Input: dimensioned drawing with shaded views. Units: mm. Origin: part minimum x, y, z. Round coordinates to 2 decimals unless told otherwise and drop trailing zeros. Loops run counter-clockwise (first coordinate to the right, second up) from the corner with the lowest first, then second, coordinate; pieces in that order, holes last. Notation, with made-up numbers: (52, -12) - (77, -12) arc R19 ccw to (77, 17) - close; hole circle Ø8 at (18.25, 67.25). An arc over 180 degrees is marked (long way). One line per question, with ' | ' between items.
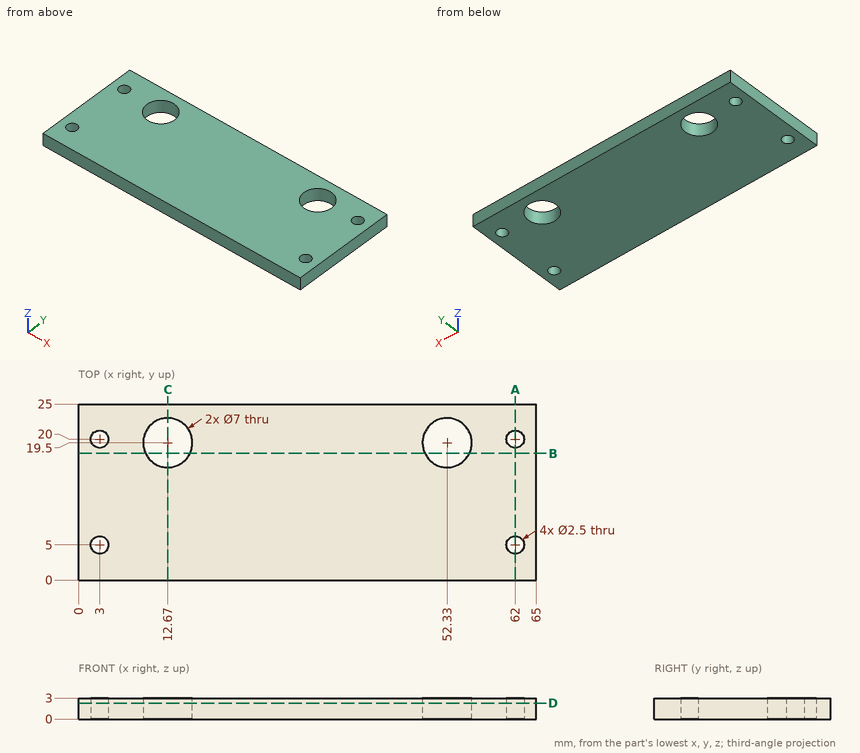
1. Material intervals for probe 1 along Y at (x, z) = (62, 1.55); probe 2 along Y at (x, z) = (12.67, 0.8); probe 3 along X at (y, z) = (16.5, 0.95), sorted ascending.
Worked out:
probe 1: y = 0 to 3.75, 6.25 to 18.75, 21.25 to 25 | probe 2: y = 0 to 16, 23 to 25 | probe 3: x = 0 to 10.87, 14.47 to 50.53, 54.13 to 65
2. Section query B-B, the plane y = 18. Return loops of the section in (x, z).
Worked out:
outline: (0, 0) - (9.51, 0) - (9.51, 3) - (0, 3) - close; (15.83, 0) - (49.17, 0) - (49.17, 3) - (15.83, 3) - close; (55.49, 0) - (65, 0) - (65, 3) - (55.49, 3) - close
3. Section query C-C, the plane x = 12.67. Return loops of the section in (y, z), plus the area to 3 significant figures.
Worked out:
outline: (0, 0) - (16, 0) - (16, 3) - (0, 3) - close; (23, 0) - (25, 0) - (25, 3) - (23, 3) - close | area: 54.0 mm2
4. Section query A-A, the plane x = 62. Return loops of the section in (y, z), plus the area to 3 significant figures.
Worked out:
outline: (0, 0) - (3.75, 0) - (3.75, 3) - (0, 3) - close; (6.25, 0) - (18.75, 0) - (18.75, 3) - (6.25, 3) - close; (21.25, 0) - (25, 0) - (25, 3) - (21.25, 3) - close | area: 60.0 mm2
5. Section query D-D, the plane z = 2.3. Return loops of the section in (x, y), plus the area to 3 significant figures.
Worked out:
outline: (0, 0) - (65, 0) - (65, 25) - (0, 25) - close; hole circle Ø2.5 at (3, 5); hole circle Ø2.5 at (3, 20); hole circle Ø7 at (12.67, 19.5); hole circle Ø7 at (52.33, 19.5); hole circle Ø2.5 at (62, 5); hole circle Ø2.5 at (62, 20) | area: 1,530 mm2
